```python
from build123d import *

# Parameters (mm, degrees)
SKETCH1_W           = 12.5
SKETCH1_H           = 30
BOSS_EXTRUDE1_DEPTH = 5
SKETCH2_W           = 12.5
SKETCH2_H           = 19.6
BOSS_EXTRUDE2_DEPTH = 2
SKETCH3_R           = 2.1
CUT_EXTRUDE1_DEPTH  = 15
SKETCH4_R           = 1.6
CUT_EXTRUDE2_DEPTH  = 10
LPATTERN1_COUNT     = 2
LPATTERN1_PITCH     = 7.5


with BuildPart() as part:
    # Sketch1 → Boss-Extrude1 (new body)
    with BuildSketch(Plane(origin=(0, 0, 0), x_dir=(1, 0, 0), z_dir=(0, 1, 0))):
        with Locations((6.25, 15)):
            Rectangle(SKETCH1_W, SKETCH1_H)
    extrude(amount=BOSS_EXTRUDE1_DEPTH)

    # Sketch2 → Boss-Extrude2 (add)
    with BuildSketch(Plane.XZ):
        with Locations((6.25, -15)):
            Rectangle(SKETCH2_W, SKETCH2_H)
    extrude(amount=BOSS_EXTRUDE2_DEPTH)

    # Sketch3 → Cut-Extrude1 (cut)
    with BuildSketch(Plane.ZY):
        with Locations((-19.8, 2.5)):
            Circle(SKETCH3_R)
        with Locations((-9.8, 2.5)):
            Circle(SKETCH3_R)
    extrude(amount=-CUT_EXTRUDE1_DEPTH, mode=Mode.SUBTRACT)

    # Sketch4 → Cut-Extrude2 (cut)
    with BuildSketch(Plane(origin=(0, 5, 0), x_dir=(1, 0, 0), z_dir=(0, 1, 0))):
        with Locations((2.5, 27.5)):
            Circle(SKETCH4_R)
        with Locations((2.5, 2.5)):
            Circle(SKETCH4_R)
    cut_extrude2 = extrude(amount=-CUT_EXTRUDE2_DEPTH, mode=Mode.SUBTRACT)

    # LPattern1: Cut-Extrude2 ×2
    with Locations(*[(i * LPATTERN1_PITCH, 0, 0) for i in range(1, LPATTERN1_COUNT)]):
        add(cut_extrude2, mode=Mode.SUBTRACT)


solid = part.part
```
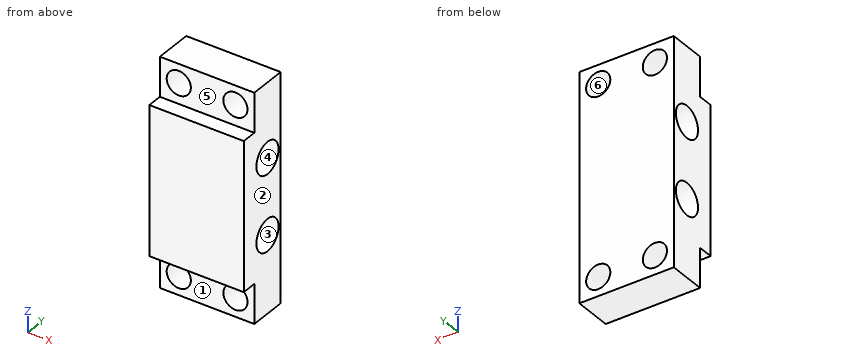
For this review, take the finished solid that the model builds, in its own axes (mm). Face numbers are marked on the shaded views. A direction names the side the tool comes from. Coordinates: 2 decimals unless noted, no trailing zeros. Loops run counter-clockwise (first coordinate to the right, second up) from the corner with the lowest first, then second, coordinate; pieces in that order, holes last.
1. Add section A-A, the plane x = 2.5. Give the boundary of the cut face in (y, z).
2. Add section B-B, the plane z = -19.8. Give the boundary of the cut face in (x, y).
3. For line 1 (X direction, y = 3.4, z = -27.5); line 2 (Z direction, x = 2.5, y = 2.35); line 3 (Y direction, x = 4.5, z = -9.8), list the stretches that pass through material, from the lowest coordinate up.
4. Add section C-C, the plane y = 3.75. Give the boundary of the cut face in (x, z).
5. Add section D-D, the plane x = 6.5. Give the boundary of the cut face in (y, z).
6. For the marked faces 1 and 2, list the 3-axis set-ups (+Z, -Z, +X, -X, +Y, -Y) from which the entire face can be reached by the end or side of a thin tool; tool diameter is ignored.
7. Mouldability with a two-part tool opening along Y and no side actions: class the marked faces 3, 4, 5 and 6 as +Y half, -Y half, draft (parallel to the pull), parting line (faces both ways), or undercut.
8. Insertion check: P1, Ø0.6, axis at x = 8, y = -0.5, coming from the +Z side; P2, Ø2.5, axis at x = 2.5, z = -2.5, coming from the +Y side; P3, Ø4, axis at x = 8, z = -2.5, coming from the -Y side; P4, Ø0.6, axis at x = 5, y = -1, coming from the -Z side. Each pin has a flat end and moves straight along its axis. Give the tip position at first contact, or say it passes through.
Result:
1. outline: (-2, -24.8) - (0, -24.8) - (0, -25.9) - (5, -25.9) - (5, -4.1) - (0, -4.1) - (0, -5.2) - (-2, -5.2) - close; (0, -30) - (5, -30) - (5, -29.1) - (0, -29.1) - close; (0, -0.9) - (5, -0.9) - (5, 0) - (0, 0) - close; hole circle Ø4.2 at (2.5, -19.8); hole circle Ø4.2 at (2.5, -9.8)
2. outline: (0, -2) - (12.5, -2) - (12.5, 0.4) - (0, 0.4) - close; (0, 4.6) - (12.5, 4.6) - (12.5, 5) - (0, 5) - close
3. line 1: x = 0 to 0.9, 4.1 to 8.4, 11.6 to 12.5
3. line 2: z = -30 to -29.1, -25.9 to -21.89, -17.71 to -11.89, -7.71 to -4.1, -0.9 to 0
3. line 3: y = -2 to 0.4, 4.6 to 5
4. outline: (0, -30) - (12.5, -30) - (12.5, -21.49) - (0, -21.49) - close; (0, -18.11) - (12.5, -18.11) - (12.5, -11.49) - (0, -11.49) - close; (0, -8.11) - (12.5, -8.11) - (12.5, 0) - (0, 0) - close; hole circle Ø3.2 at (2.5, -27.5); hole circle Ø3.2 at (2.5, -2.5); hole circle Ø3.2 at (10, -27.5); hole circle Ø3.2 at (10, -2.5)
5. outline: (-2, -24.8) - (0, -24.8) - (0, -30) - (5, -30) - (5, 0) - (0, 0) - (0, -5.2) - (-2, -5.2) - close; hole circle Ø4.2 at (2.5, -19.8); hole circle Ø4.2 at (2.5, -9.8)
6. face 1: -Z, +X, -X, -Y
6. face 2: +Z, -Z, +X, +Y, -Y
7. face 3: undercut
7. face 4: undercut
7. face 5: -Y half
7. face 6: draft
8. P1: stops at z = -5.2
8. P2: passes through
8. P3: stops at y = 0
8. P4: stops at z = -24.8
